Print and shaded views of the part. All mm, measured from the part's lowest x, y and z. A direction names the side the tool comes from. Round coordinates to 2 decimals unless told otherwise and drop trailing zeros. Order: outer loops, then holes, each group sorted by start corner. A loop starts at its lowest first (then second) coordinate and runs counter-clockwise, first axis right, second up. Notation, with made-up numbers: M 14.25,-20 L 71.25,-20 A21 cw 71.25,-16 Z; hole C 20.5,-3.5 d4. An arc over 180 degrees is marked long. Use CSV: the item, a comma, the result in double quotes.
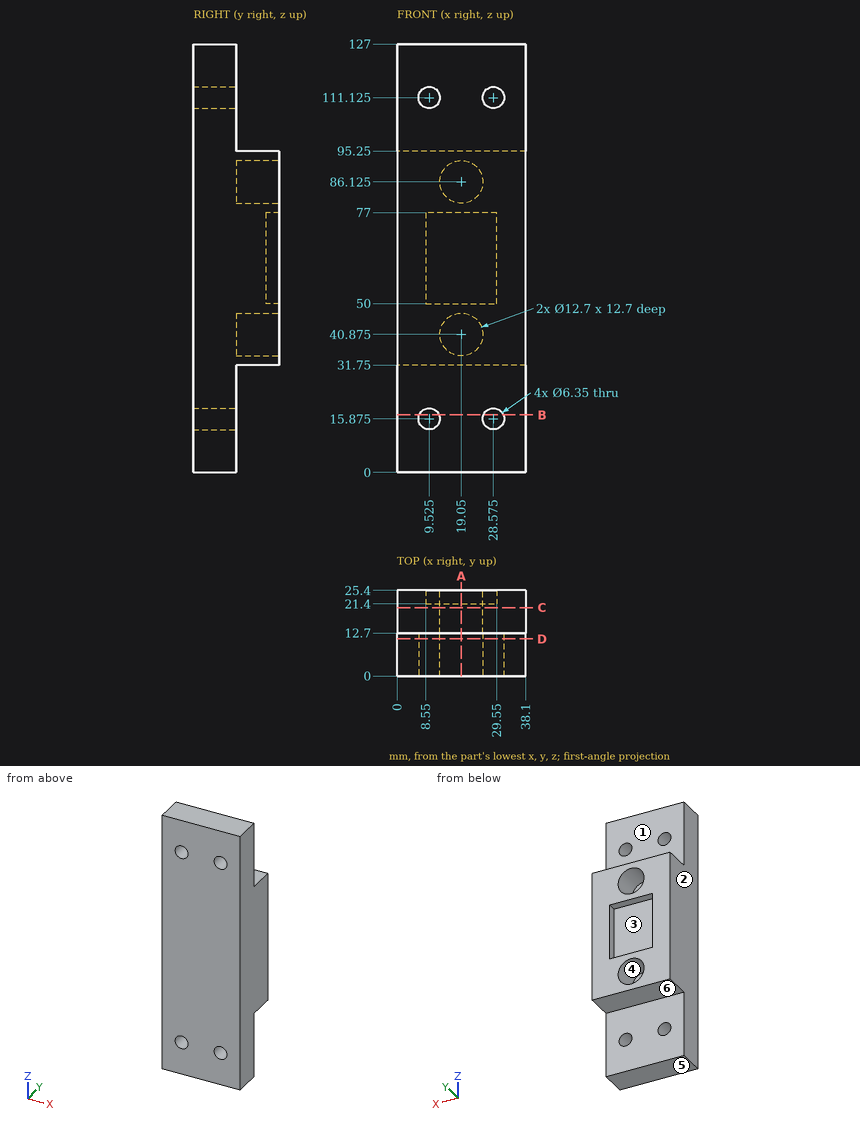
(1) Two-plate mould, pull along X, no slides. Class the marked faces 1, 2 and 3: released by +X, released by -X, zero draft, split by the parting line, or undercut.
Answer block:
face 1,"zero draft"
face 2,"released by -X"
face 3,"undercut"
(2) Cut at B-B, the plane z = 17. Give the cut face in (x, y), and give its area (3 significant figures).
Answer block:
outline,"M 0,0 L 6.56,0 L 6.56,12.7 L 0,12.7 Z; M 12.49,0 L 25.61,0 L 25.61,12.7 L 12.49,12.7 Z; M 31.54,0 L 38.1,0 L 38.1,12.7 L 31.54,12.7 Z"
area,"333 mm²"
(3) Drop flat-ended pins along their axis: pin 1 (16 mm diameter, centred on x = 18.5, z = 117, fed in from +Y); pin 2 (10 mm diameter, centred on x = 12, y = 19, fed in from -Z); pin 3 (2 mm diameter, centred on x = 24, y = 24, fed in from +Z); pin 4 (5.5 mm diameter, centred on x = 28.575, z = 15.875, fed in from -Y). Give the stop position or say it passes through.
Answer block:
pin 1,"stops at y = 12.7"
pin 2,"stops at z = 31.75"
pin 3,"stops at z = 95.25"
pin 4,"passes through"
(4) Cut at A-A, the plane x = 19.05. Give the cut face in (y, z) (3 decimals), and give its area (3 significant figures).
Answer block:
outline,"M 0,0 L 12.7,0 L 12.7,31.75 L 25.4,31.75 L 25.4,34.525 L 12.7,34.525 L 12.7,47.225 L 25.4,47.225 L 25.4,50 L 21.4,50 L 21.4,77 L 25.4,77 L 25.4,79.775 L 12.7,79.775 L 12.7,92.475 L 25.4,92.475 L 25.4,95.25 L 12.7,95.25 L 12.7,127 L 0,127 Z"
area,"1,990 mm²"
(5) Cut at D-D, the plane y = 11. Give the cut face in (x, z) (3 decimals), and give its area (3 significant figures).
Answer block:
outline,"M 0,0 L 38.1,0 L 38.1,127 L 0,127 Z; hole C 9.525,15.875 d6.35; hole C 9.525,111.125 d6.35; hole C 28.575,15.875 d6.35; hole C 28.575,111.125 d6.35"
area,"4,710 mm²"
(6) Cut at C-C, the plane y = 20.25. Give the cut face in (x, z) (3 decimals), and give its area (3 significant figures).
Answer block:
outline,"M 0,31.75 L 38.1,31.75 L 38.1,95.25 L 0,95.25 Z; hole C 19.05,40.875 d12.7; hole C 19.05,86.125 d12.7"
area,"2,170 mm²"
(7) Tool access for the marked faces 4, 5 and 6: list every direction of +Z, -Z, +X, -X, +Y, -Y with a clear straight run to the whole face (end or side of a thin tool).
Answer block:
face 4,"+Y"
face 5,"-Z, +X, -X, +Y, -Y"
face 6,"-Z, +X, -X, +Y"
(8) Wall check: line 1 (Z direction, x = 19.05, y = 17) (3 decimals); line 2 (Z direction, x = 19.5, y = 22.75); line 3 (X direction, y = 1.5, z = 111). Give the ranges that are in metal, low to high. Write a range as from..to.
Answer block:
line 1,"z = 31.75..34.525, 47.225..79.775, 92.475..95.25"
line 2,"z = 31.75..34.54, 47.21..50, 77..79.79, 92.46..95.25"
line 3,"x = 0..6.35, 12.7..25.4, 31.75..38.1"
